from build123d import *

# Parameters (mm, degrees)
SKETCH1_R           = 14
BOSS_EXTRUDE1_DEPTH = 34
SKETCH2_R           = 18.5
BOSS_EXTRUDE2_DEPTH = 23
SKETCH3_R           = 6
BOSS_EXTRUDE3_DEPTH = 6
SKETCH5_R           = 2.75
BOSS_EXTRUDE4_DEPTH = 15
CUT_EXTRUDE1_DEPTH  = 12
SKETCH7_R           = 13.875
BOSS_EXTRUDE5_DEPTH = 3


with BuildPart() as part:
    # Sketch1 → Boss-Extrude1 (new body)
    with BuildSketch(Plane(origin=(0, 0, 0), x_dir=(0, 0, -1), z_dir=(1, 0, 0))):
        Circle(SKETCH1_R)
    extrude(amount=-BOSS_EXTRUDE1_DEPTH)

    # Sketch2 → Boss-Extrude2 (add)
    with BuildSketch(Plane.ZY.offset(34)):
        Circle(SKETCH2_R)
    extrude(amount=BOSS_EXTRUDE2_DEPTH)

    # Sketch3 → Boss-Extrude3 (add)
    with BuildSketch(Plane.ZY.offset(57)):
        with Locations((-6.8, 0)):
            Circle(SKETCH3_R)
    extrude(amount=BOSS_EXTRUDE3_DEPTH)

    # Sketch5 → Boss-Extrude4 (add)
    with BuildSketch(Plane.ZY.offset(63)):
        with Locations((-6.8, 0)):
            Circle(SKETCH5_R)
    extrude(amount=BOSS_EXTRUDE4_DEPTH)

    # Sketch6 → Cut-Extrude1 (cut)
    with BuildSketch(Plane.ZY.offset(78)):
        with BuildLine():
            Line((-8.55, 2.121320344), (-5.05, 2.121320344))
            ThreePointArc((-5.05, 2.121320344), (-6.8, 2.75), (-8.55, 2.121320344))
        make_face()
    extrude(amount=-CUT_EXTRUDE1_DEPTH, mode=Mode.SUBTRACT)

    # Sketch7 → Boss-Extrude5 (add)
    with BuildSketch(Plane(origin=(0, 0, 0), x_dir=(0, 0, -1), z_dir=(1, 0, 0))):
        Circle(SKETCH7_R)
    extrude(amount=BOSS_EXTRUDE5_DEPTH)


solid = part.part
Source: CAD feature listing. Evaluate the final solid. Frame: model axes, mm. A direction names the side the tool comes from. Coordinates: 2 decimals unless noted, no trailing zeros. Loops run counter-clockwise (first coordinate to the right, second up) from the corner with the lowest first, then second, coordinate; pieces in that order, holes last. Notation, with made-up numbers: (70.25, -24.75) - (94.25, -24.75) arc R9 ccw to (94.25, -13.75) - close; hole circle Ø9 at (54, -4.75). An arc over 180 degrees is marked (long way). One line per item, written item: value. Start each with the question number.
1. Section A-A (z = 0). Return the cut outline in (x, y) (3 decimals).
2. Section D-D (y = -7). Return the cut outline in (x, z).
3. Ray query, L1, parallel to X at y = 4, z = -9.5; L2, parallel to X at y = -6.5, z = -1; L3, parallel to Z at x = -68, y = 0. Return the intervals inside material, ascending.
4. Contact query for flat-ended pins moving along their axis: P1, Ø12, axis at x = -40, y = -10, coming from the -Z side; P2, Ø12, axis at x = -39, y = 3.5, coming from the -Z side; P3, Ø6, axis at x = -49.5, y = -14.5, coming from the -Z side; P4, Ø0.5, axis at y = 2.5, z = -7, coming from the -X side. Output: stop coordinate, or through.
5. Section C-C (x = -32). Return the cut outline in (y, z).
6. Section B-B (y = 0). Return the cut outline in (x, z) (3 decimals).
7. Set-up query: faces 1 (the cylindrical face through (-59.96, -3.65, -11.56)), 2 (the cylindrical face through (-16.762, -5.362, -12.932)), 3 (the cylindrical face through (-45.34, -18.06, -4.01)), 4 (the flat face through (-72, 2.121, -7)), 5 (the flat face through (3, 0, 0)). Return all of +Z, -Z, +X, -X, +Y, -Y with unobstructed straight access to the full face (end or side cutting, diameter ignored); none if empty.
Verdict:
1. outline: (-57, -18.5) - (-34, -18.5) - (-34, -14) - (0, -14) - (0, -13.875) - (3, -13.875) - (3, 13.875) - (0, 13.875) - (0, 14) - (-34, 14) - (-34, 18.5) - (-57, 18.5) - close
2. outline: (-57, -17.12) - (-34, -17.12) - (-34, -12.12) - (0, -12.12) - (0, -11.98) - (3, -11.98) - (3, 11.98) - (0, 11.98) - (0, 12.12) - (-34, 12.12) - (-34, 17.12) - (-57, 17.12) - close
3. L1: x = -63 to 3
3. L2: x = -57 to 3
3. L3: z = -9.55 to -4.05
4. P1: stops at z = -18.06
4. P2: stops at z = -18.5
4. P3: stops at z = -14.49
4. P4: stops at x = -66
5. outline: circle Ø28 at (0, 0)
6. outline: (-78, -9.55) - (-63, -9.55) - (-63, -12.8) - (-57, -12.8) - (-57, -18.5) - (-34, -18.5) - (-34, -14) - (0, -14) - (0, -13.875) - (3, -13.875) - (3, 13.875) - (0, 13.875) - (0, 14) - (-34, 14) - (-34, 18.5) - (-57, 18.5) - (-57, -0.8) - (-63, -0.8) - (-63, -4.05) - (-78, -4.05) - close
7. face 1: -X
7. face 2: +X
7. face 3: +X, -X
7. face 4: +Z, -Z, -X, +Y
7. face 5: +Z, -Z, +X, +Y, -Y
